Input: part model. Units: mm. Frame: model coordinates. A direction names the side the tool comes from. Round coordinates to 2 decimals unless told otherwise and drop trailing zeros. Loops run counter-clockwise (first coordinate to the right, second up) from the corner with the lowest first, then second, coordinate; pieces in that order, holes last. Notation, with made-up numbers: (54.5, -30) - (68.5, -30) arc R7 cw to (68.5, -23) - close; hole circle Ø8 at (-38.5, -3). An arc over 180 degrees is marked (long way). One line per question, with ' | ' between items. Start each with the question number.
Item 1: First-contact query: pin 1 (6 mm diameter, centred on x = 18, y = 0, fed in from +Z); pin 2 (1 mm diameter, centred on y = 2, z = 6.5, fed in from +X); pin 3 (5 mm diameter, centred on x = -5.5, z = 7, fed in from -Y). Flat tips, straight axial feed; report the tip coordinate or a pass-through.
Item 2: Section C-C, the plane x = 0. Return loops of the section in (y, z), plus the area to 3 significant figures.
Item 3: Draft query along Y for faces 3 (the face through (24, 0, 2)), 4 (the face through (-15, 1, 4)), 5 (the face through (20.528, 0.796, 2.028)). Return one class per face: pulls with the +Y half, pulls with the -Y half, needs draft (parallel to the pull), parting line crosses it, or undercut.
Item 4: Section B-B, the plane z = 2. Return loops of the section in (x, y) (3 decimals).
Item 5: Section D-D, the plane y = -8. Return loops of the section in (x, z), plus the area to 3 significant figures.
Item 6: Set-up query: faces 1 (the face through (5, -10, 8.5)), 2 (the face through (15, -1, 4)). Return all of +Z, -Z, +X, -X, +Y, -Y with unobstructed straight access to the full face (end or side cutting, diameter ignored); none if empty.
Item 7: Material intervals for line 1 along Y through (x, z) = (2.5, 1.5); line 2 along X through (y, z) = (5.25, 4.5); line 3 along X through (y, z) = (-7.75, 5.75), sorted ascending.
Item 8: Section A-A, the plane y = 0. Return loops of the section in (x, z).
```python
from build123d import *

# Parameters (mm, degrees)
BASE_SKETCH_R                     = 11
BASE_EXTRUDE_DEPTH                = 4
BEARING_RETAINING_RING_SKETCH_R   = 13.5
BEARING_RETAINING_RING_SKETCH_R_2 = 11
BEARING_RETAINING_RING_DEPTH      = 8.5
MOUNTING_HOLES_D                  = 5.3


with BuildPart() as part:
    # Base Sketch → Base Extrude (new body)
    with BuildSketch(Plane.XY):
        with BuildLine():
            Line((-20.5, 5.454356057), (-5.625, 12.272301129))
            ThreePointArc((-5.625, 12.272301129), (0, 13.5), (5.625, 12.272301129))
            Line((5.625, 12.272301129), (20.5, 5.454356057))
            ThreePointArc((20.5, 5.454356057), (24, 0), (20.5, -5.454356057))
            Line((20.5, -5.454356057), (5.625, -12.272301129))
            ThreePointArc((5.625, -12.272301129), (0, -13.5), (-5.625, -12.272301129))
            Line((-5.625, -12.272301129), (-20.5, -5.454356057))
            ThreePointArc((-20.5, -5.454356057), (-24, 0), (-20.5, 5.454356057))
        make_face()
        Circle(BASE_SKETCH_R, mode=Mode.SUBTRACT)
    extrude(amount=BASE_EXTRUDE_DEPTH)

    # Bearing Retaining Ring Sketch → Bearing Retaining Ring (add)
    with BuildSketch(Plane.XY):
        with Locations(Location((0, 0, 0), (0, 0, 114.624318352))):
            Circle(BEARING_RETAINING_RING_SKETCH_R)
        Circle(BEARING_RETAINING_RING_SKETCH_R_2, mode=Mode.SUBTRACT)
    extrude(amount=BEARING_RETAINING_RING_DEPTH)

    # Mounting Holes (through all)
    with Locations(Plane(origin=(0, 0, 0), x_dir=(-1, 0, 0), z_dir=(0, 0, -1))):
        with Locations((18, 0), (-18, 0)):
            Hole(MOUNTING_HOLES_D / 2)


solid = part.part
```
Return value:
1) pin 1: z = 4 | pin 2: x = 13.42 | pin 3: y = -13.16
2) outline: (-13.5, 0) - (-11, 0) - (-11, 8.5) - (-13.5, 8.5) - close; (11, 0) - (13.5, 0) - (13.5, 8.5) - (11, 8.5) - close | area: 42.5 mm2
3) face 3: parting line crosses it | face 4: needs draft | face 5: undercut
4) outline: (-20.5, -5.454) - (-5.625, -12.272) arc R13.5 ccw to (5.625, -12.272) - (20.5, -5.454) arc R6 ccw to (20.5, 5.454) - (5.625, 12.272) arc R13.5 ccw to (-5.625, 12.272) - (-20.5, 5.454) arc R6 ccw to start; hole circle Ø5.3 at (-18, 0); hole circle Ø22 at (0, 0); hole circle Ø5.3 at (18, 0)
5) outline: (-14.95, 0) - (-7.55, 0) - (-7.55, 8.5) - (-10.87, 8.5) - (-10.87, 4) - (-14.95, 4) - close; (7.55, 0) - (14.95, 0) - (14.95, 4) - (10.87, 4) - (10.87, 8.5) - (7.55, 8.5) - close | area: 89.1 mm2
6) face 1: +Z, +X, -X, +Y, -Y | face 2: +Z, +X
7) line 1: -13.27 to -10.71, 10.71 to 13.27 | line 2: -12.44 to -9.67, 9.67 to 12.44 | line 3: -11.05 to -7.81, 7.81 to 11.05
8) outline: (-24, 0) - (-20.65, 0) - (-20.65, 4) - (-24, 4) - close; (-15.35, 0) - (-11, 0) - (-11, 8.5) - (-13.5, 8.5) - (-13.5, 4) - (-15.35, 4) - close; (11, 0) - (15.35, 0) - (15.35, 4) - (13.5, 4) - (13.5, 8.5) - (11, 8.5) - close; (20.65, 0) - (24, 0) - (24, 4) - (20.65, 4) - close
